```python
from build123d import *

# Parameters (mm, degrees)
BOSS_EXTRUDE1_DEPTH = 58.42
CHAMFER5_START      = -95.906013746
CHAMFER5_OUTLINE_W  = 100
CHAMFER5_OUTLINE_H  = 58.42
CHAMFER5_DEPTH      = 45.787595784


with BuildPart() as part:
    # Sketch1 → Boss-Extrude1 (new body)
    with BuildSketch(Plane(origin=(0, 0, 0), x_dir=(1, 0, 0), z_dir=(0, 1, 0))):
        with BuildLine():
            Line((-66.673768512, 0), (-37.067821873, 47.633329988))
            ThreePointArc((-37.067821873, 47.633329988), (-11.329209284, 68.541566023), (21.82652777, 69.113940477))
            Line((21.82652777, 69.113940477), (53.138492197, 58.903517294))
            Line((53.138492197, 58.903517294), (0, -77.45185891))
            Line((0, -77.45185891), (-66.673768512, -77.45185891))
            Line((-66.673768512, -77.45185891), (-66.673768512, 0))
        make_face()
    extrude(amount=BOSS_EXTRUDE1_DEPTH)

    # Chamfer4
    # the kernel refuses this chamfer: 25.4 mm, written as the material it takes off along each edge
    with BuildSketch(Plane(origin=(53.138492197, -68.954815123, -58.903517294), x_dir=(-0.9507298394814789, 0, -0.3100205998309166), z_dir=(0, 1, 0))) as chamfer4_piece_1:
        with BuildLine():
            Line((27.572040722, -0.738386759), (0.816641802, 27.56983389))
            Line((0.816641802, 27.56983389), (0.309449153, 27.598462833))
            ThreePointArc((0.309449153, 27.598462833), (0.269734882, 13.792739557), (-0.507192649, 0.028628943))
            Line((-0.507192649, 0.028628943), (0, -0.508))
            ThreePointArc((0, -0.508), (13.786020361, -0.508), (27.572040722, -1.246386759))
            Line((27.572040722, -1.246386759), (27.572040722, -0.738386759))
        make_face()
    extrude(amount=196.329630245, mode=Mode.SUBTRACT)

    # Chamfer5: read off the stored shape, not the designer's step
    # Chamfer5 outline → Chamfer5 (cut)
    with BuildSketch(Plane(origin=(0, 0, 0), x_dir=(0.48585842778436206, 0, 0.8740375210200692), z_dir=(0.8740375210200692, 0, -0.48585842778436206)).offset(CHAMFER5_START)):
        with Locations((12, -29.21)):
            Rectangle(CHAMFER5_OUTLINE_W, CHAMFER5_OUTLINE_H)
    extrude(amount=CHAMFER5_DEPTH, mode=Mode.SUBTRACT)


solid = part.part
```
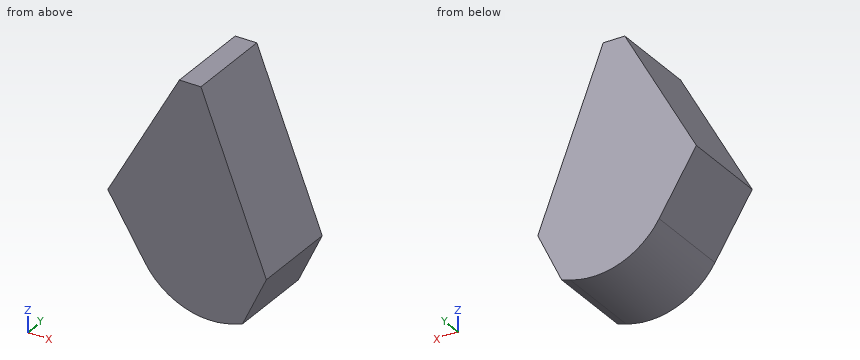
Source: CAD feature listing. Evaluate the final solid. Frame: model axes, mm. Give positions to 0.01 mm unless a question says otherwise; leave off trailing zeros. Loops run counter-clockwise (first coordinate to the right, second up) from the corner with the lowest first, then second, coordinate; pieces in that order, holes last. Notation, with made-up numbers: (73.25, 62) - (82.25, 62) arc R18 ccw to (82.25, 76) - close; hole circle Ø3 at (33, 55.25). An arc over 180 degrees is marked (long way). Use CSV: the item, a comma, the result in double quotes.
1) Line query: line 1 (Z direction, x = -45.5, y = 35.5); line 2 (Z direction, x = -9.5, y = 32.5); line 3 (X direction, y = 27, z = 60.5). Output: solid intervals per line, ascending.
Worked out:
line 1,"z = -34.07 to 21.3"
line 2,"z = -69.17 to 77.45"
line 3,"x = -23.71 to 6.61"
2) Cut plane A-A (y = 44). Output: boundary loops of the cut face in (x, z).
Worked out:
outline,"(-61.75, -7.93) - (-37.07, -47.63) arc R50.8 ccw to (21.83, -69.11) - (27.59, -67.24) - (43.38, -33.86) - (0, 77.45) - (-14.29, 77.45) - close"
3) Pin query (flat end, axial travel): P1, Ø12, axis at y = 8, z = 5, coming from the -X side; P2, Ø4, axis at x = -18.5, y = 32, coming from the -Z side; P3, Ø6, axis at x = -29, y = 13.5, coming from the -Z side. Return the tip coordinate at first contact, or that it passes through.
Worked out:
P1,"stops at x = -57.9"
P2,"stops at z = -66.32"
P3,"stops at z = -60.21"
4) Cut plane B-B (x = -16). Output: boundary loops of the cut face in (y, z), and give its area (3 significant figures).
Worked out:
outline,"(0, -66.57) - (58.42, -66.57) - (58.42, 74.37) - (0, 74.37) - close"
area,"8,230 mm^2"
5) Cut plane C-C (z = 29). Output: boundary loops of the cut face in (x, y), and give its area (3 significant figures).
Worked out:
outline,"(-41.22, 0) - (18.88, 0) - (18.88, 58.42) - (-41.22, 58.42) - close"
area,"3,510 mm^2"
